from build123d import *

# Parameters (mm, degrees)
F0_R     = 72.39
F0_R_2   = 2.159
F0_R_3   = 12.065
F1_DEPTH = 25.4


with BuildPart() as f1:
    # F0 (on Front) → F1 (new body)
    with BuildSketch(Plane.XZ):
        Circle(F0_R)
        with Locations((-30.340522, -52.551325)):
            Circle(F0_R_2, mode=Mode.SUBTRACT)
        with BuildLine():
            ThreePointArc((0, -54.938267), (-9.259687, -54.12592), (-18.262741, -51.813624))
            ThreePointArc((-18.262741, -51.813624), (-22.13476, -48.031833), (-21.684225, -42.638179))
            Line((-21.684225, -42.638179), (-14.554108, -30.288454))
            ThreePointArc((-14.554108, -30.288454), (-12.88956, -28.892127), (-10.7169, -28.893036))
            ThreePointArc((-10.7169, -28.893036), (-5.441359, -30.321806), (0, -30.835938))
            ThreePointArc((0, -30.835938), (5.441359, -30.321806), (10.7169, -28.893036))
            ThreePointArc((10.7169, -28.893036), (12.88956, -28.892127), (14.554108, -30.288454))
            Line((14.554108, -30.288454), (21.684225, -42.638179))
            ThreePointArc((21.684225, -42.638179), (22.13476, -48.031833), (18.262741, -51.813624))
            ThreePointArc((18.262741, -51.813624), (9.259687, -54.12592), (0, -54.938267))
        make_face(mode=Mode.SUBTRACT)
        with BuildLine():
            ThreePointArc((-47.577935, -27.469134), (-51.504265, -19.043836), (-54.003286, -10.090814))
            ThreePointArc((-54.003286, -10.090814), (-52.664168, -4.846652), (-47.767859, -2.54))
            Line((-47.767859, -2.54), (-33.507625, -2.54))
            ThreePointArc((-33.507625, -2.54), (-31.466096, -3.283378), (-30.380553, -5.16541))
            ThreePointArc((-30.380553, -5.16541), (-28.980133, -10.448548), (-26.704705, -15.417969))
            ThreePointArc((-26.704705, -15.417969), (-23.538775, -19.873258), (-19.663653, -23.727626))
            ThreePointArc((-19.663653, -23.727626), (-18.576536, -25.60875), (-18.953516, -27.748454))
            Line((-18.953516, -27.748454), (-26.083634, -40.09818))
            ThreePointArc((-26.083634, -40.09818), (-30.529407, -43.185181), (-35.740544, -41.72281))
            ThreePointArc((-35.740544, -41.72281), (-42.244578, -35.082084), (-47.577935, -27.469134))
        make_face(mode=Mode.SUBTRACT)
        with Locations((-11.90625, -20.62223)):
            Circle(F0_R_2, mode=Mode.SUBTRACT)
        with Locations((30.340522, -52.551325)):
            Circle(F0_R_2, mode=Mode.SUBTRACT)
        with Locations((11.90625, -20.62223)):
            Circle(F0_R_2, mode=Mode.SUBTRACT)
        with BuildLine():
            ThreePointArc((47.577935, -27.469134), (42.244578, -35.082084), (35.740544, -41.72281))
            ThreePointArc((35.740544, -41.72281), (30.529407, -43.185181), (26.083634, -40.09818))
            Line((26.083634, -40.09818), (18.953516, -27.748454))
            ThreePointArc((18.953516, -27.748454), (18.576536, -25.60875), (19.663653, -23.727626))
            ThreePointArc((19.663653, -23.727626), (23.538775, -19.873258), (26.704705, -15.417969))
            ThreePointArc((26.704705, -15.417969), (28.980133, -10.448548), (30.380553, -5.16541))
            ThreePointArc((30.380553, -5.16541), (31.466096, -3.283378), (33.507625, -2.54))
            Line((33.507625, -2.54), (47.767859, -2.54))
            ThreePointArc((47.767859, -2.54), (52.664168, -4.846652), (54.003286, -10.090814))
            ThreePointArc((54.003286, -10.090814), (51.504265, -19.043836), (47.577935, -27.469134))
        make_face(mode=Mode.SUBTRACT)
        with Locations((-60.681044, 0)):
            Circle(F0_R_2, mode=Mode.SUBTRACT)
        with BuildLine():
            ThreePointArc((-47.577935, 27.469134), (-42.244578, 35.082084), (-35.740544, 41.72281))
            ThreePointArc((-35.740544, 41.72281), (-30.529407, 43.185181), (-26.083634, 40.09818))
            Line((-26.083634, 40.09818), (-18.953516, 27.748454))
            ThreePointArc((-18.953516, 27.748454), (-18.576536, 25.60875), (-19.663653, 23.727626))
            ThreePointArc((-19.663653, 23.727626), (-23.538775, 19.873258), (-26.704705, 15.417969))
            ThreePointArc((-26.704705, 15.417969), (-28.980133, 10.448548), (-30.380553, 5.16541))
            ThreePointArc((-30.380553, 5.16541), (-31.466096, 3.283378), (-33.507625, 2.54))
            Line((-33.507625, 2.54), (-47.767859, 2.54))
            ThreePointArc((-47.767859, 2.54), (-52.664168, 4.846652), (-54.003286, 10.090814))
            ThreePointArc((-54.003286, 10.090814), (-51.504265, 19.043836), (-47.577935, 27.469134))
        make_face(mode=Mode.SUBTRACT)
        with Locations((-23.8125, 0)):
            Circle(F0_R_2, mode=Mode.SUBTRACT)
        with Locations((-11.90625, 20.62223)):
            Circle(F0_R_2, mode=Mode.SUBTRACT)
        with Locations((-30.340522, 52.551325)):
            Circle(F0_R_2, mode=Mode.SUBTRACT)
        Circle(F0_R_3, mode=Mode.SUBTRACT)
        with Locations((23.8125, 0)):
            Circle(F0_R_2, mode=Mode.SUBTRACT)
        with Locations((11.90625, 20.62223)):
            Circle(F0_R_2, mode=Mode.SUBTRACT)
        with Locations((60.681044, 0)):
            Circle(F0_R_2, mode=Mode.SUBTRACT)
        with BuildLine():
            ThreePointArc((47.577935, 27.469134), (51.504265, 19.043836), (54.003286, 10.090814))
            ThreePointArc((54.003286, 10.090814), (52.664168, 4.846652), (47.767859, 2.54))
            Line((47.767859, 2.54), (33.507625, 2.54))
            ThreePointArc((33.507625, 2.54), (31.466096, 3.283378), (30.380553, 5.16541))
            ThreePointArc((30.380553, 5.16541), (28.980133, 10.448548), (26.704705, 15.417969))
            ThreePointArc((26.704705, 15.417969), (23.538775, 19.873258), (19.663653, 23.727626))
            ThreePointArc((19.663653, 23.727626), (18.576536, 25.60875), (18.953516, 27.748454))
            Line((18.953516, 27.748454), (26.083634, 40.09818))
            ThreePointArc((26.083634, 40.09818), (30.529407, 43.185181), (35.740544, 41.72281))
            ThreePointArc((35.740544, 41.72281), (42.244578, 35.082084), (47.577935, 27.469134))
        make_face(mode=Mode.SUBTRACT)
        with BuildLine():
            ThreePointArc((14.554108, 30.288454), (12.88956, 28.892127), (10.7169, 28.893036))
            ThreePointArc((10.7169, 28.893036), (5.441359, 30.321806), (0, 30.835938))
            ThreePointArc((0, 30.835938), (-5.441359, 30.321806), (-10.7169, 28.893036))
            ThreePointArc((-10.7169, 28.893036), (-12.88956, 28.892127), (-14.554108, 30.288454))
            Line((-14.554108, 30.288454), (-21.684225, 42.638179))
            ThreePointArc((-21.684225, 42.638179), (-22.13476, 48.031833), (-18.262741, 51.813624))
            ThreePointArc((-18.262741, 51.813624), (-9.259687, 54.12592), (0, 54.938267))
            ThreePointArc((0, 54.938267), (9.259687, 54.12592), (18.262741, 51.813624))
            ThreePointArc((18.262741, 51.813624), (22.13476, 48.031833), (21.684225, 42.638179))
            Line((21.684225, 42.638179), (14.554108, 30.288454))
        make_face(mode=Mode.SUBTRACT)
        with Locations((30.340522, 52.551325)):
            Circle(F0_R_2, mode=Mode.SUBTRACT)
    extrude(amount=F1_DEPTH)


solid = f1.part
For this review, take the finished solid that the model builds, in its own axes (mm). Round coordinates to 2 decimals unless told otherwise and drop trailing zeros. Write each loop counter-clockwise with the first axis right and the second up, starting at its lowest first coordinate (ties: lowest second). Pieces come first, ordered by that corner, then holes. Notation, with made-up numbers: (73, 20.25) - (121, 20.25) arc R17 ccw to (121, 40.25) - close; hole circle Ø11 at (84.5, 23). An arc over 180 degrees is marked (long way). Write item = value, one per line. Start each with the question number.
1. Draft analysis for pull direction X (two halves, no side actions). For faces 1 (the face through (-1, -25.4, -15)), 2 (the face through (23.49, -12.52, -19.93)), state which applies: released by +X, released by -X, zero draft, split by the parting line, or undercut.
2. Wall thickness on L1, parallel to Z at x = -0.5, y = -1.25; L2, parallel to Z at x = 35.5, y = -4.75; L3, parallel to Z at x = -17.5, y = -6: over which ranges is each line inside the solid? List them lowest first.
3. Consider section C-C on x = 42. State the section outline as (y, z) points, plus the area to 3 significant figures.
4. Consider section B-B on x = -60.5. State the section outline as (y, z) points.
5. For pin 1 Ø4 at (x, z) = (60.68, 0) entering from -Y; pin 2 Ø1.5 at (x, y) = (21.5, -10.5) entering from -Z; pin 3 Ø7 at (x, z) = (-30.34, -52.55) entering from -Y; pin 4 Ø4.5 at (x, y) = (43, -7.5) entering from +Z, all flat-tipped, find the tip position at first contact; note any pin that passes through.
6. Consider section D-D on y = -8. Give the number of separate pieces and of enclosed holes in the cut face, plus the area to 3 significant figures.
7. Consider section A-A on z = 0. State the section outline as (x, y) points (1 decimal), plus the area to 3 significant figures.
Evaluation:
q1.face_1 = zero draft
q1.face_2 = undercut
q2.L1 = -72.39 to -54.93, -30.83 to -12.05, 12.05 to 30.83, 54.93 to 72.39
q2.L2 = -63.09 to -41.92, -2.54 to 2.54, 41.92 to 63.09
q2.L3 = -70.24 to -52.07, -35.39 to 35.39, 52.07 to 70.24
q3.outline = (-25.4, -58.96) - (0, -58.96) - (0, -35.37) - (-25.4, -35.37) - close; (-25.4, -2.54) - (0, -2.54) - (0, 2.54) - (-25.4, 2.54) - close; (-25.4, 35.37) - (0, 35.37) - (0, 58.96) - (-25.4, 58.96) - close
q3.area = 1,330 mm2
q4.outline = (-25.4, -39.75) - (0, -39.75) - (0, -2.15) - (-25.4, -2.15) - close; (-25.4, 2.15) - (0, 2.15) - (0, 39.75) - (-25.4, 39.75) - close
q5.pin_1 = through
q5.pin_2 = -69.35
q5.pin_3 = -25.4
q5.pin_4 = 59.83
q6.separate_pieces = 1
q6.enclosed_holes = 19
q6.area = 10,200 mm2
q7.outline = (-72.4, -25.4) - (-62.8, -25.4) - (-62.8, 0) - (-72.4, 0) - close; (-58.5, -25.4) - (-26, -25.4) - (-26, 0) - (-58.5, 0) - close; (-21.7, -25.4) - (-12.1, -25.4) - (-12.1, 0) - (-21.7, 0) - close; (12.1, -25.4) - (21.7, -25.4) - (21.7, 0) - (12.1, 0) - close; (26, -25.4) - (58.5, -25.4) - (58.5, 0) - (26, 0) - close; (62.8, -25.4) - (72.4, -25.4) - (72.4, 0) - (62.8, 0) - close
q7.area = 2,630 mm2
